The figure shows three views and two pictorial views of one solid part (mm, origin at its lowest corner). Answer the questions. Give positions to 0.01 mm unless a question says otherwise; leave off trailing zeros. Loops run counter-clockwise (first coordinate to the right, second up) from the corner with the lowest first, then second, coordinate; pieces in that order, holes last. Notation, with made-up numbers: M 69,-14 L 102,-14 A27 ccw 102,21 Z; hole C 18.5,49 d8. An arc over 180 degrees is marked long. Write item = value, one per line. Start each with the question number.
1. Section D-D on z = 0.3 is taken. Determine the outline of the cut face in (x, y).
2. The mould has two halves that part along X. Classify the marked faces 1, 2 and 3: released by +X, released by -X, zero draft, split by the parting line, or undercut.
3. Consider L1, parallel to X at y = 8.25, z = 0.4; L2, parallel to Y at x = 7.5, z = 1.2; L3, parallel to X at y = 0.75, z = 0.9. Determine where each line is inside the solid, lowest interval first. Write a range as [from, to].
4. Section C-C on y = 1.5 is taken. Determine the outline of the cut face in (x, z), plus the area to 3 significant figures.
5. Section A-A on x = 7.5 is taken. Determine the outline of the cut face in (y, z), plus the area to 3 significant figures.
6. Flat-ended cylindrical pins translate along their axes: pin 1 Ø2.5 at (x, y) = (13.5, 7.5) entering from +Z; pin 2 Ø1.6 at (x, y) = (1.5, 7.5) entering from +Z. Find the tip coordinate at first contact, or state that the pin passes through.
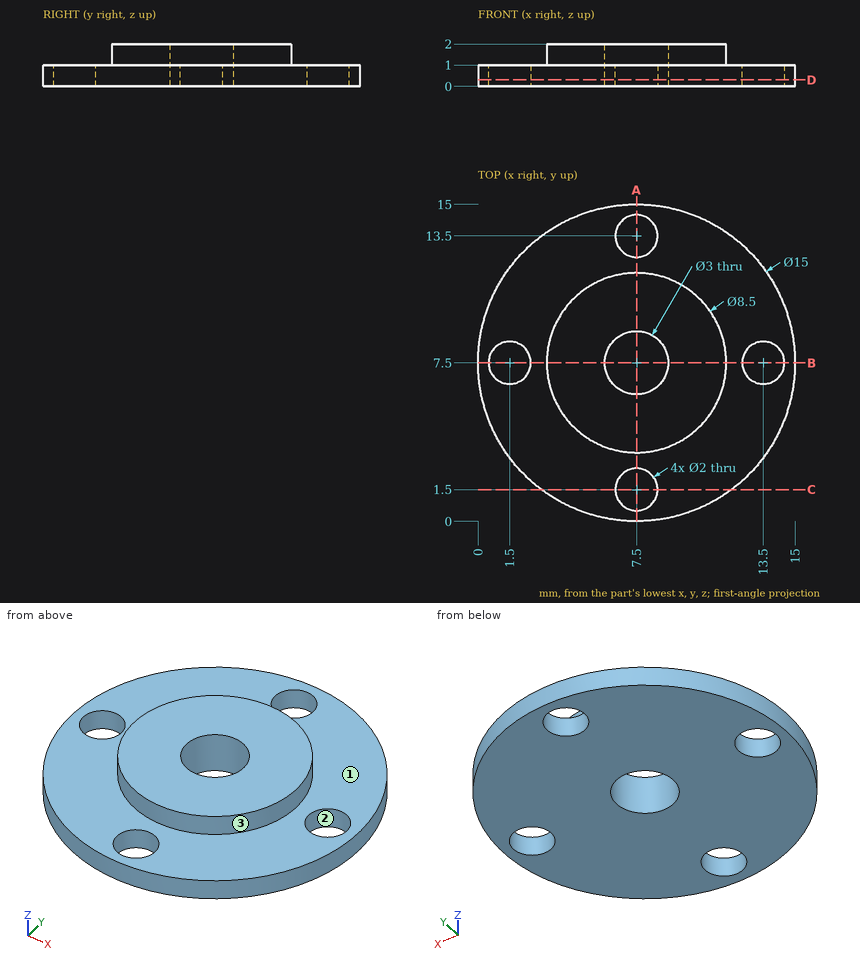
Verdict:
q1.outline = C 7.5,7.5 d15; hole C 1.5,7.5 d2; hole C 7.5,7.5 d3; hole C 7.5,1.5 d2; hole C 7.5,13.5 d2; hole C 13.5,7.5 d2
q2.face_1 = zero draft
q2.face_2 = undercut
q2.face_3 = split by the parting line
q3.L1 = [0.04, 0.84], [2.16, 6.2], [8.8, 12.84], [14.16, 14.96]
q3.L2 = [3.25, 6], [9, 11.75]
q3.L3 = [4.23, 6.84], [8.16, 10.77]
q4.outline = M 3,0 L 6.5,0 L 6.5,1 L 3,1 Z; M 8.5,0 L 12,0 L 12,1 L 8.5,1 Z
q4.area = 7.00 mm2
q5.outline = M 0,0 L 0.5,0 L 0.5,1 L 0,1 Z; M 2.5,0 L 6,0 L 6,2 L 3.25,2 L 3.25,1 L 2.5,1 Z; M 9,0 L 12.5,0 L 12.5,1 L 11.75,1 L 11.75,2 L 9,2 Z; M 14.5,0 L 15,0 L 15,1 L 14.5,1 Z
q5.area = 13.5 mm2
q6.pin_1 = 1
q6.pin_2 = through
